```python
from build123d import *

# Parameters (mm, degrees)
ESQUISSE1_R      = 3
ESQUISSE1_R_2    = 1
EXTRUSION1_DEPTH = 5


with BuildPart() as part:
    # Esquisse1 → Extrusion1 (new body)
    with BuildSketch(Plane.XY):
        with BuildLine():
            Line((52.730599116, -2.952254244), (7.830086245, -0.723670796))
            ThreePointArc((7.830086245, -0.723670796), (3.699182558, -2.567602385), (2.746849637, -6.989989861))
            Line((2.746849637, -6.989989861), (12.746849637, -44.989989861))
            ThreePointArc((12.746849637, -44.989989861), (16.307085805, -48.552192625), (21.161053557, -47.209223095))
            Line((21.161053557, -47.209223095), (56.061566429, -11.437806542))
            ThreePointArc((56.061566429, -11.437806542), (57.136985769, -6.119100628), (52.730599116, -2.952254244))
        make_face()
        with Locations((7.582222324, -5.717523364)):
            Circle(ESQUISSE1_R, mode=Mode.SUBTRACT)
        with Locations((52.482735195, -7.946106812)):
            Circle(ESQUISSE1_R, mode=Mode.SUBTRACT)
        with Locations((17.582222324, -43.717523364)):
            Circle(ESQUISSE1_R, mode=Mode.SUBTRACT)
        with Locations((24.216673772, -19.733908354)):
            Circle(ESQUISSE1_R_2, mode=Mode.SUBTRACT)
    extrude(amount=EXTRUSION1_DEPTH)


solid = part.part
```
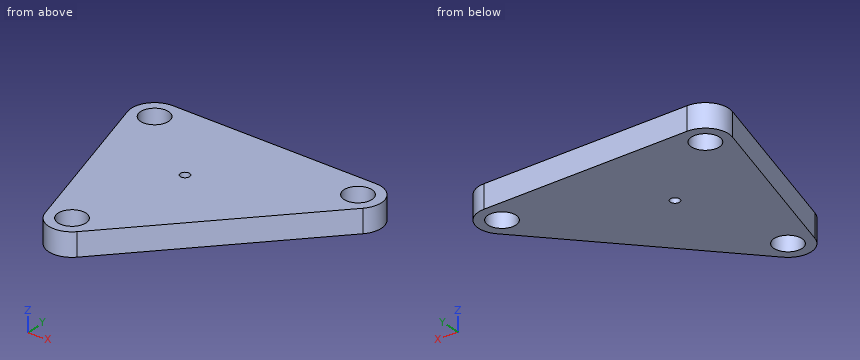
Source: CAD feature listing. Evaluate the final solid. Frame: model axes, mm. Round coordinates to 2 decimals unless told otherwise and drop trailing zeros. Loops run counter-clockwise (first coordinate to the right, second up) from the corner with the lowest first, then second, coordinate; pieces in that order, holes last. Notation, with made-up numbers: (34, 71) - (89, 71) arc R23 cw to (89, 98) - close; hole circle Ø2 at (17.25, 49). An arc over 180 degrees is marked (long way). Use CSV: the item, a comma, the result in double quotes.
Q1. Pin query (flat end, axial travel): pin 1 Ø3 at (y, z) = (-41.5, 2) entering from -X; pin 2 Ø5 at (x, y) = (7.58, -5.72) entering from +Z; pin 3 Ø1 at (x, z) = (18.5, 1) entering from +Y. Return the tip coordinate at first contact, or that it passes through.
Reported:
pin 1,"x = 11.43"
pin 2,"through"
pin 3,"y = -1.23"
Q2. Section query A-A, the plane z = 2.8. Output: boundary loops of the cut face in (x, y), then the cut area to 3 significant figures.
Reported:
outline,"(2.75, -6.99) - (12.75, -44.99) arc R5 ccw to (21.16, -47.21) - (56.06, -11.44) arc R5 ccw to (52.73, -2.95) - (7.83, -0.72) arc R5 ccw to start; hole circle Ø6 at (7.58, -5.72); hole circle Ø6 at (17.58, -43.72); hole circle Ø2 at (24.22, -19.73); hole circle Ø6 at (52.48, -7.95)"
area,"1,500 mm^2"
Q3. Section query C-C, the plane x = 47. Output: boundary loops of the cut face in (y, z), then the cut area to 3 significant figures.
Reported:
outline,"(-20.73, 0) - (-2.67, 0) - (-2.67, 5) - (-20.73, 5) - close"
area,"90.3 mm^2"
Q4. Section query B-B, the plane y = -18. Output: boundary loops of the cut face in (x, z).
Reported:
outline,"(5.64, 0) - (49.66, 0) - (49.66, 5) - (5.64, 5) - close"
Q5. Ray query, line 1 along Y through (x, z) = (16, 1.95); line 2 along Y through (x, z) = (50, 2.05); line 3 along X through (y, z) = (-42, 2.8). Return the intervals inside material, ascending.
Reported:
line 1,"-48.46 to -46.27, -41.17 to -1.13"
line 2,"-17.65 to -9.63, -6.26 to -2.82"
line 3,"11.96 to 15.12, 20.04 to 26.24"
